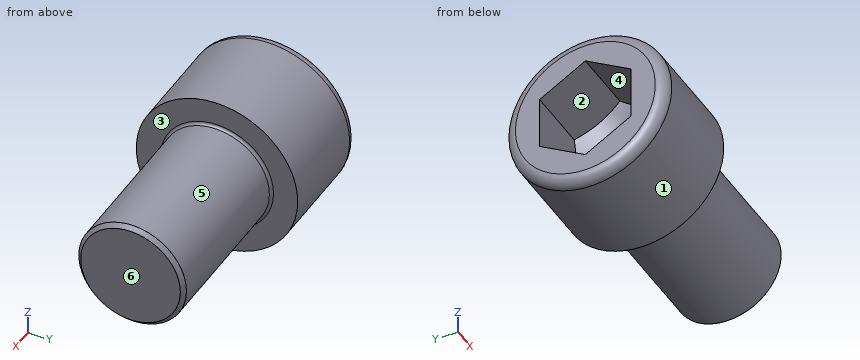
Autodesk Inventor part; units mm, degrees
ref_plane "Work Plane1" through (29, 0, 0) normal (0, -1, 0) x (1, 0, 0)
ref_plane "YZ Plane" through (0, 0, 0) normal (1, 0, 0) x (0, 1, 0)
ref_plane "XZ Plane" through (0, 0, 0) normal (0, 1, 0) x (-1, 0, 0)
sketch "Skizze1" plane through (0, 0, 0) normal (0, 0, 1) x (1, 0, 0)
  line L0 (-11.6667, 0) -> (150, 0)
  line L1 (150, 0) -> (150, 50)
  line L2 (150, 50) -> (15, 50)
  line L3 (15, 50) -> (11.3192, 50)
  line L4 (11.3192, 50) -> (0, 50)
  line L5 (0, 50) -> (0, 75)
  line L6 (0, 75) -> (-100, 75)
  line L7 (-100, 75) -> (-100, 49.0748)
  line L8 (-100, 49.0748) -> (-40, 49.0748)
  line L9 (-40, 49.0748) -> (-11.6667, 0)
  line L10 (-150, 0) -> (200, 0)
  line L11 (0, -15) -> (0, 90)
  line L12 (15, 50) -> (0, 50) construction
  dimension "d1" = 135
  dimension "d2" = 3.6808
  dimension "d3" = 100
  dimension "d4" = 60
  dimension "d5" = 60
  dimension "d6" = 100
  dimension "d7" = 100
  dimension "d8" = 98.1496
  dimension "d9" = 150
  dimension "d26" = 150
revolve "Körper" add sketch "Skizze1" angle 360 about axis through (-11.6667, 0, 0) along (1, 0, 0)
sketch "Skizze2" plane through (-100, 0, 0) normal (-1, 0, 0) x (0, 0, 1)
  circle A0 centre (0, 0) radius 49.0748
  line L0 (0, -105) -> (0, 105)
  line L1 (-105, 0) -> (105, 0)
  line L2 (49.0748, 0) -> (24.5374, -42.5)
  line L3 (24.5374, -42.5) -> (-24.5374, -42.5)
  line L4 (-24.5374, -42.5) -> (-49.0748, 0)
  line L5 (-49.0748, 0) -> (-24.5374, 42.5)
  line L6 (-24.5374, 42.5) -> (24.5374, 42.5)
  line L7 (24.5374, 42.5) -> (49.0748, 0)
extrude "Loch" add sketch "Skizze2" against normal up to next contours L7 A0 | A0 L2 | L6 L0 A0 | A0 L0 L3 | L0 L6 A0 | A0 L3 L0 | L4 A0 | A0 L5
fillet "Rundung1" radius 10 1 edges at (-100, -75, 0)
thread "Gewinde"
chamfer "Fase1" distance 3.6807 distance2 3.6807 1 edges at (150, -50, 0) measured on face at (150, -3.2515, 16.3464)
ref_plane "Work Plane1" through (29, 0, 0) normal (0, -1, 0) x (1, 0, 0)
fillet "Fillet2" radius 2.5 1 edges at (0, -50, 0)
equation "\"d1\" = GEL"
equation "\"d3\" = KOH"
equation "\"d4\" = INTI"
equation "\"d6\" = GD"
equation "\"d7\" = BDM"
equation "\"d8\" = 1.1547 * SW"
equation "\"d9\" = KOD"
equation "\"d26\" = NLG"
equation "\"d30\" = R"
equation "\"d17\" = RR"
equation "\"d13\" = GEL"
equation "\"d15\" = -0.5 * SPD + 0.5 * GD"
equation "\"d16\" = GUL"
equation "\"GD\" = NND"
equation "\"NLG\" = 150"
equation "\"GEL\" = 135"
equation "\"KOD\" = 150"
equation "\"KOH\" = 100"
equation "\"INTI\" = 60"
equation "\"GAL\" = 0.61345 * PTC"
equation "\"GUL\" = 0.61345 * PTC"
equation "\"BDM\" = NND"
equation "\"SW\" = 85"
equation "\"SPD\" = NND - 1.2269 * PTC"
equation "\"R\" = 2.5"
equation "\"TOA\" = 30deg"
equation "\"GD1\" = THREADDIA - 1.2269 * PTC"
equation "\"FAWI\" = 45deg"
equation "\"ANG\" = 120deg"
equation "\"PTC\" = 6"
equation "\"E0\" = 1.155 * SW"
properties part number "DIN 912 - M100 x 6 x 150" material "Stahl, weich"
CAD build for the part. Positions are in the model's coordinates, mm. Face numbers are marked on the shaded views. A direction names the side the tool comes from. Round coordinates to 2 decimals unless told otherwise and drop trailing zeros. Write each loop counter-clockwise with the first axis right and the second up, starting at its lowest first coordinate (ties: lowest second). Pieces come first, ordered by that corner, then holes. Notation, with made-up numbers: (50, -14) - (95, -14) arc R20 ccw to (95, 2) - close; hole circle Ø2 at (62.25, 65). An arc over 180 degrees is marked (long way). Write item = value, one per line. Start each with the question number.
Q1. Band-saw the part on C-C (x = 44). Give the cut face in (y, z), then the cut area to 3 significant figures.
Q2. Mould opens along Z. For the marked faces 1, 2 and 3 say: pulls with the +Z half, pulls with the -Z half, needs draft (parallel to the pull), parting line crosses it, or undercut.
Q3. Drop flat-ended pins along their axis: pin 1 (1 mm diameter, centred on x = 122, y = -39.5, fed in from -Z); pin 2 (8 mm diameter, centred on x = 67.5, z = 12, fed in from +Y); pin 3 (3 mm diameter, centred on x = -16.5, y = 46, fed in from -Z). Give the stop position or say it passes through.
Q4. Band-saw the part on B-B (x = -32.5). Give the cut face in (y, z), then the cut area to 3 significant figures.
Q5. Probe L1, parallel to X at y = 38, z = -48; L2, parallel to Z at x = -73, y = 8; L3, parallel to Y at x = -68, z = 16. List the from-to ranges inside material, lowest first. Write a range as from..to.
Q6. Which spindle directions (+Z, -Z, +X, -X, +Y, -Y) get a long thin tool onto all of the face, cutting with end or side? Do the marked faces 4, 5 and 6. Say none if no direction does.
Q7. Band-saw the part on A-A (x = -4). Give the cut face in (y, z).
Answers below:
q1.outline = circle Ø100 at (0, 0)
q1.area = 7,850 mm2
q2.face_1 = parting line crosses it
q2.face_2 = undercut
q2.face_3 = needs draft
q3.pin_1 = -31.29
q3.pin_2 = 49.36
q3.pin_3 = -60.37
q4.outline = circle Ø150 at (0, 0); hole circle Ø72.17 at (0, 0)
q4.area = 13,600 mm2
q5.L1 = -100..0
q5.L2 = -74.57..-44.46, 44.46..74.57
q5.L3 = -73.27..-42.5, 42.5..73.27
q6.face_4 = -X
q6.face_5 = +X
q6.face_6 = +Z, -Z, +X, +Y, -Y
q7.outline = circle Ø150 at (0, 0)
